Input: dimensioned drawing with shaded views. Units: mm. Origin: part minimum x, y, z. Give positions to 0.01 mm unless a question says otherwise; leave off trailing zeros. Order: outer loops, then holes, each group sorted by start corner. A loop starts at its lowest first (then second) coordinate and runs counter-clockwise, first axis right, second up.
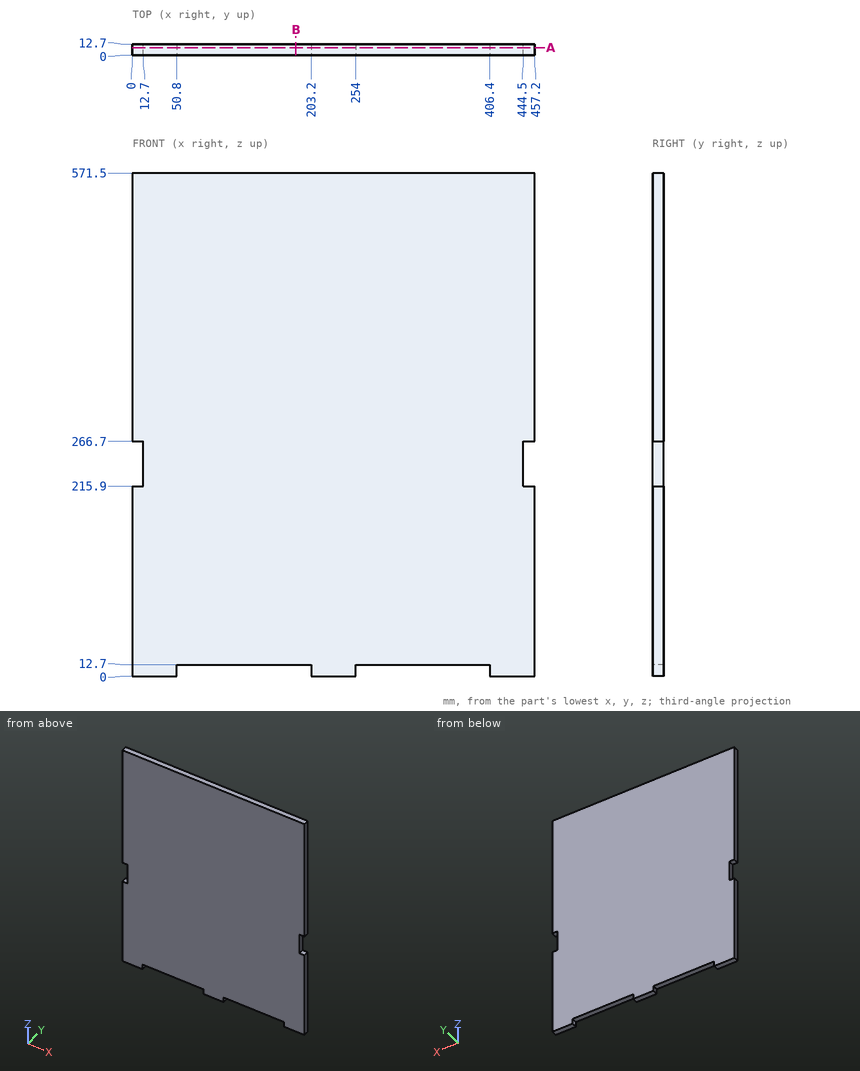
1) Cut plane B-B (x = 186). Return the cut outline in (y, z), then the cut area to 3 significant figures.
2) Line query: probe 1 along X at (y, z) = (3, 260); probe 2 along Z at (x, y) = (357, 7). Output: solid intervals per line, ascending.
3) First-contact query: P1, Ø6, axis at y = 4.5, z = 264.5, coming from the +X side; P2, Ø4, axis at x = 309.5, y = 6, coming from the -Z side. Flat tips, straight axial feed; report the tip coordinate or a pass-through.
4) Cut plane A-A (y = 8.5). Return the cut outline in (x, z), then the cut area to 3 significant figures.
Geometry says:
1. outline: (0, 12.7) - (12.7, 12.7) - (12.7, 571.5) - (0, 571.5) - close
1. area: 7,100 mm2
2. probe 1: x = 12.7 to 444.5
2. probe 2: z = 12.7 to 571.5
3. P1: stops at x = 457.2
3. P2: stops at z = 12.7
4. outline: (0, 0) - (50.8, 0) - (50.8, 12.7) - (203.2, 12.7) - (203.2, 0) - (254, 0) - (254, 12.7) - (406.4, 12.7) - (406.4, 0) - (457.2, 0) - (457.2, 215.9) - (444.5, 215.9) - (444.5, 266.7) - (457.2, 266.7) - (457.2, 571.5) - (0, 571.5) - (0, 266.7) - (12.7, 266.7) - (12.7, 215.9) - (0, 215.9) - close
4. area: 256,000 mm2
